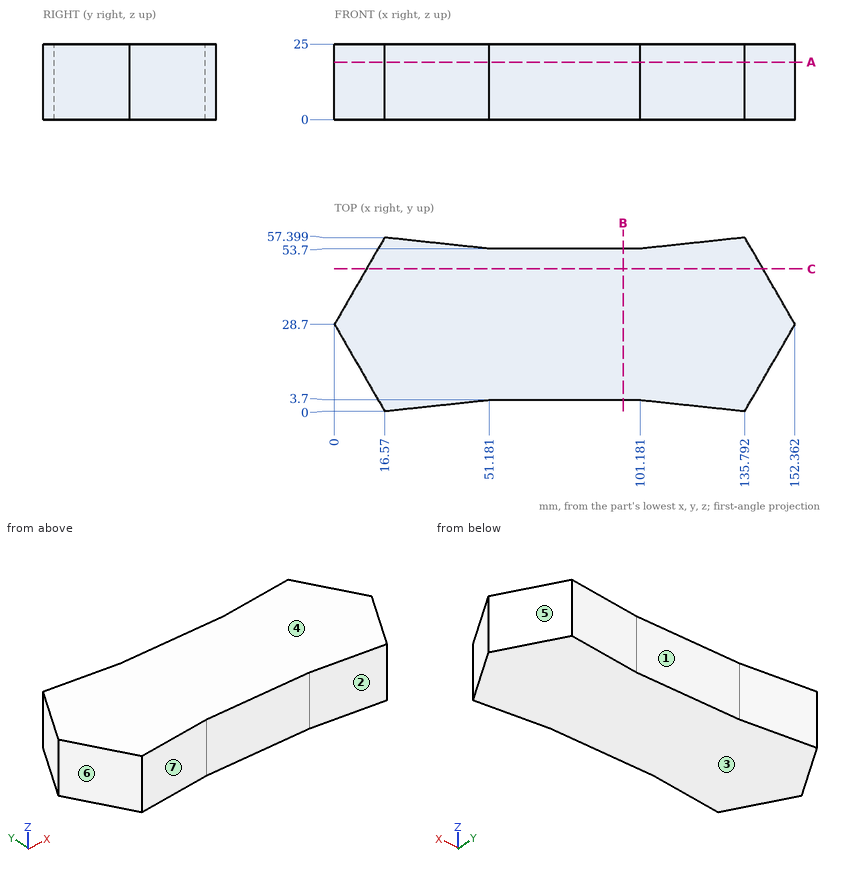
Could you check a few things on this drawing? It's one solid part, dimensions in mm from its lowest x, y, z. A direction names the side the tool comes from. Round coordinates to 2 decimals unless told otherwise and drop trailing zeros. Order: outer loops, then holes, each group sorted by start corner. A loop starts at its lowest first (then second) coordinate and runs counter-clockwise, first axis right, second up.
Q1. Imagine slicing it at C-C, the plane y = 47. List the corners of the cut face in (x, z) for me (1 decimal), then the cut area to 3 significant figures.
Geometry says:
outline: (10.6, 0) - (141.8, 0) - (141.8, 25) - (10.6, 25) - close
area: 3,280 mm2
Q2. Please list where these lines run through material, in increasing order: probe 1 along Y at (x, z) = (97, 9.75); probe 2 along Y at (x, z) = (122, 19.75) (1 decimal); probe 3 along X at (y, z) = (36, 4) (1 decimal).
Geometry says:
probe 1: y = 3.7 to 53.7
probe 2: y = 1.5 to 55.9
probe 3: x = 4.2 to 148.1
Q3. Imagine slicing it at B-B, the plane x = 95.5. List the corners of the cut face in (y, z) for me, then the cut area to 3 significant figures.
Geometry says:
outline: (3.7, 0) - (53.7, 0) - (53.7, 25) - (3.7, 25) - close
area: 1,250 mm2
Q4. Which directions (+Z, -Z, +X, -X, +Y, -Y) give clear straight access to the entire face, cutting with the end or side of a thin tool? Please do the marked faces 1, 2 and 3.
Geometry says:
face 1: +Z, -Z, +Y
face 2: +Z, -Z, -Y
face 3: -Z, +X, -X, +Y, -Y
Q5. Imagine slicing it at A-A, the plane z = 19. List the corners of the cut face in (x, y) for me, then the cut area to 3 significant figures.
Geometry says:
outline: (0, 28.7) - (16.57, 0) - (51.18, 3.7) - (101.18, 3.7) - (135.79, 0) - (152.36, 28.7) - (135.79, 57.4) - (101.18, 53.7) - (51.18, 53.7) - (16.57, 57.4) - close
area: 7,170 mm2
Q6. I'm going to push flat-ended pins straight in: P1, Ø1, axis at x = 35, z = 3, coming from the +Y side; P2, Ø1.5, axis at y = 39, z = 19.5, coming from the -X side (1 decimal); P3, Ø1.5, axis at y = 35.5, z = 5, coming from the +X side. Where does each tip first touch, or does it pass through?
Geometry says:
P1: stops at y = 55.48
P2: stops at x = 5.5
P3: stops at x = 148.87
Q7. Thinking about a two-plate mould opening in X: for the marked faces 4, 5, 6 and 7, which applies, released by +X, released by -X, zero draft, split by the parting line, or undercut?
Geometry says:
face 4: zero draft
face 5: released by +X
face 6: released by -X
face 7: undercut
